Verification items for the finished model (mm, model axes). A direction names the side the tool comes from. Coordinates: 2 decimals unless noted, no trailing zeros. Order: outer loops, then holes, each group sorted by start corner. A loop starts at its lowest first (then second) coordinate and runs counter-clockwise, first axis right, second up. Notation, with made-up numbers: (-5, 38) -> (41, 38) arc R31 ccw to (41, 63) -> close; hole circle Ø5 at (32, 49.5). An arc over 180 degrees is marked (long way). Write item = value, one per line. Start each with the question number.
1. Cross-section at D-D on z = -29. Record the cut outline in (x, y).
2. Cross-section at C-C on y = 19.5. Record the cut outline in (x, z).
3. Cross-section at A-A on x = 0. Record the cut outline in (y, z).
4. Cross-section at B-B on z = 0. Record the cut outline in (x, y), plus the area to 3 significant figures.
5. Release check for a two-part mould opening along X. For faces 1 (the cylindrical face through (-0.766, 1.972, 48.353)), 2 (the cylindrical face through (46.798, 21.692, 29.836)), 3 (the flat face through (-37, 44, 16)) record: +X half, -X half, draft (parallel to the pull), parting line (faces both ways), or undercut.
6. Set-up check for faces 4 (the flat face through (0, 4, 50)), 5 (the flat face through (1, 0, -1)): record each of +Z, -Z, +X, -X, +Y, -Y from which the full face is reachable in a straight line by a thin tool's end or side.
7. Go/stop test with flat-tipped pins: P1, Ø1, axis at x = -25, z = -37.5, coming from the +Y side; P2, Ø3, axis at y = 75, z = 15, coming from the -X side; P3, Ø4, axis at x = -11.5, z = -3.5, coming from the +Y side; P4, Ø3, axis at x = 26.5, z = -13, coming from the -Y side. Record where each tip stops, or that it passes through.
8. Thickness scan on line 1 along Y through (x, z) = (-43.5, -18.5); line 2 along X through (y, z) = (2.45, -25.1); line 3 along X through (y, z) = (2.5, 50.2). Record the ranges inside material, lowest first. Write a range as from..to.
from build123d import *

# Parameters (mm, degrees)
SKETCH1_R           = 55.5
BOSS_EXTRUDE1_DEPTH = 44
SKETCH4_R           = 2
CUT_EXTRUDE1_DEPTH  = 4


with BuildPart() as part:
    # Sketch1 → Boss-Extrude1 (new body)
    with BuildSketch(Plane(origin=(0, 0, 0), x_dir=(1, 0, 0), z_dir=(0, 1, 0))):
        with Locations(Location((0, 0, 0), (0, 0, 270))):
            Circle(SKETCH1_R)
    extrude(amount=BOSS_EXTRUDE1_DEPTH)

    # Sketch3 → Revolve1 (revolve)
    with BuildSketch(Plane.XY):
        with BuildLine():
            Line((0, 44), (-40, 44))
            ThreePointArc((-40, 44), (-28.284271247, 72.284271247), (0, 84))
            Line((0, 84), (0, 44))
        make_face()
    revolve(axis=Axis((0, 44, 0), (0, 1, 0)))

    # Sketch4 → Cut-Extrude1 (cut)
    with BuildSketch(Plane.XZ):
        with Locations(Location((0, 50.2, 0), (0, 0, 270))):
            Circle(SKETCH4_R)
        with Locations(Location((43.47447527, -25.1, 0), (0, 0, 270))):
            Circle(SKETCH4_R)
        with Locations(Location((-43.47447527, -25.1, 0), (0, 0, 270))):
            Circle(SKETCH4_R)
    extrude(amount=-CUT_EXTRUDE1_DEPTH, mode=Mode.SUBTRACT)


solid = part.part
Worked out:
q1.outline = (-47.32, 0) -> (47.32, 0) -> (47.32, 44) -> (27.55, 44) arc R27.55 ccw to (-27.55, 44) -> (-47.32, 44) -> close
q2.outline = circle Ø111 at (0, 0)
q3.outline = (0, -55.5) -> (44, -55.5) -> (44, -40) arc R40 ccw to (44, 40) -> (44, 55.5) -> (0, 55.5) -> (0, 52.2) -> (4, 52.2) -> (4, 48.2) -> (0, 48.2) -> close
q4.outline = (-55.5, 0) -> (55.5, 0) -> (55.5, 44) -> (40, 44) arc R40 ccw to (-40, 44) -> (-55.5, 44) -> close
q4.area = 7,400 mm²
q5.face_1 = undercut
q5.face_2 = parting line
q5.face_3 = draft
q6.face_4 = -Y
q6.face_5 = +Z, -Z, +X, -X, -Y
q7.P1 = 44
q7.P2 = -22.7
q7.P3 = 82.72
q7.P4 = 0
q8.line_1 = 0..44
q8.line_2 = -49.5..-45.47, -41.47..41.47, 45.47..49.5
q8.line_3 = -23.67..-2, 2..23.67
